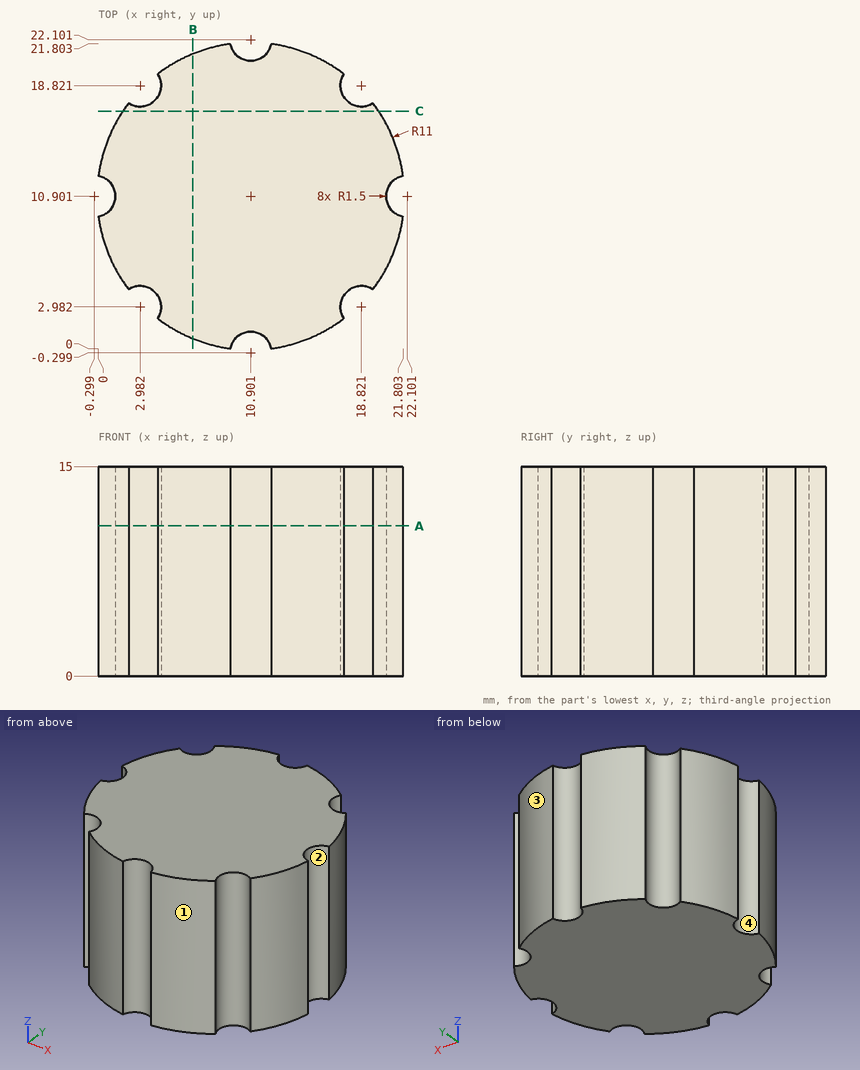
Verification items for this drawing (mm, ordinates from the low corner). Give positions to 0.01 mm unless a question says otherwise; leave off trailing zeros. Write each loop counter-clockwise with the first axis right and the second up, starting at its lowest first coordinate (ties: lowest second). Pieces come first, ordered by that corner, then holes. Notation, with made-up numbers: (30, 42.25) - (85, 42.25) arc R17 ccw to (85, 70.25) - close; hole circle Ø11 at (51, 18). An arc over 180 degrees is marked (long way). Answer as CSV lines item,"result". Start each with the question number.
1. Thickness scan on line 1 (Y direction, x = 3, z = 2.5); line 2 (X direction, y = 19.5, z = 7.5); line 3 (Y direction, x = 17.75, z = 12.75). Record the ranges inside material, lowest first.
2. Sectioned sample at A-A (z = 10.75). Record the boundary of the cut face in (x, y), then the cut area to 3 significant figures.
3. Depth check by flat-ended pin: pin 1 (1.5 mm diameter, centred on x = 14.5, y = 12.5, fed in from -Z); pin 2 (5 mm diameter, centred on x = 18.5, z = 2.5, fed in from -Y) (1 decimal); pin 3 (4 mm diameter, centred on x = 3, z = 6, fed in from +Y) (1 decimal); pin 4 (8 mm diameter, centred on x = 19, z = 12, fed in from -Y). Enter the tip coordinate at first touch or a pass-through.
4. Sectioned sample at B-B (x = 6.75). Record the boundary of the cut face in (y, z) (1 decimal), then the cut area to 3 significant figures.
5. Draft check along Y on the marked faces 1, 2, 3 and 4. Enter one of: pulls with the +Y half, pulls with the -Y half, needs draft (parallel to the pull), parting line crosses it, or undercut.
6. Sectioned sample at C-C (y = 17). Record the boundary of the cut face in (x, z), then the cut area to 3 significant figures.
Derived:
1,line 1,"4.48 to 17.32"
1,line 2,"4.32 to 17.48"
1,line 3,"4.03 to 17.77"
2,outline,"(0, 9.43) arc R11 ccw to (2.15, 4.23) arc R1.5 cw to (4.23, 2.15) arc R11 ccw to (9.43, 0) arc R1.5 cw to (12.37, 0) arc R11 ccw to (17.57, 2.15) arc R1.5 cw to (19.65, 4.23) arc R11 ccw to (21.8, 9.43) arc R1.5 cw to (21.8, 12.37) arc R11 ccw to (19.65, 17.57) arc R1.5 cw to (17.57, 19.65) arc R11 ccw to (12.37, 21.8) arc R1.5 cw to (9.43, 21.8) arc R11 ccw to (4.23, 19.65) arc R1.5 cw to (2.15, 17.57) arc R11 ccw to (0, 12.37) arc R1.5 cw to start"
2,area,"357 mm²"
3,pin 1,"z = 0"
3,pin 2,"y = 1.2"
3,pin 3,"y = 20.2"
3,pin 4,"y = 0.69"
4,outline,"(0.7, 0) - (21.1, 0) - (21.1, 15) - (0.7, 15) - close"
4,area,"306 mm²"
5,face 1,"pulls with the -Y half"
5,face 2,"undercut"
5,face 3,"pulls with the +Y half"
5,face 4,"undercut"
6,outline,"(1.75, 0) - (20.06, 0) - (20.06, 15) - (1.75, 15) - close"
6,area,"275 mm²"
